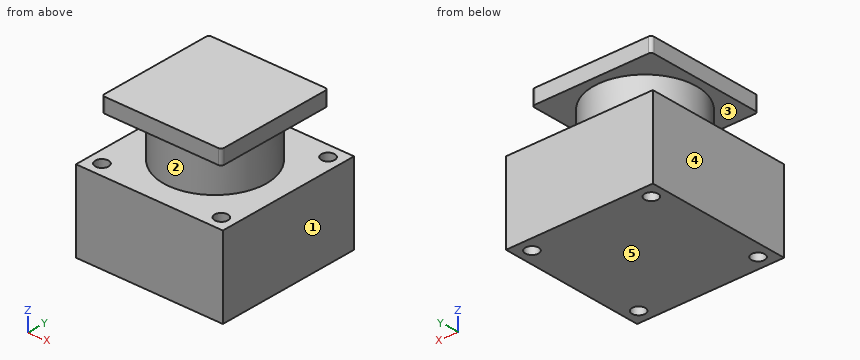
```python
from build123d import *

# Parameters (mm, degrees)
SKETCH_1_W      = 100
SKETCH_1_H      = 100
SKETCH_1_R      = 4.5
EXTRUDE_1_DEPTH = 55
SKETCH_2_R      = 35
EXTRUDE_2_DEPTH = 30
SKETCH_3_W      = 81.317279836
SKETCH_3_H      = 81.317279836
EXTRUDE_3_DEPTH = 10
FILLET_1_R      = 2


with BuildPart() as part:
    # 草图1 → 凸台-拉伸1 (new body)
    with BuildSketch(Plane.XY):
        Rectangle(SKETCH_1_W, SKETCH_1_H)
        with Locations((-40.658639918, 40.658639918)):
            Circle(SKETCH_1_R, mode=Mode.SUBTRACT)
        with Locations((40.658639918, 40.658639918)):
            Circle(SKETCH_1_R, mode=Mode.SUBTRACT)
        with Locations((40.658639918, -40.658639918)):
            Circle(SKETCH_1_R, mode=Mode.SUBTRACT)
        with Locations((-40.658639918, -40.658639918)):
            Circle(SKETCH_1_R, mode=Mode.SUBTRACT)
    extrude(amount=EXTRUDE_1_DEPTH)

    # 草图2 → 凸台-拉伸2 (add)
    with BuildSketch(Plane.XY.offset(55)):
        Circle(SKETCH_2_R)
    extrude(amount=EXTRUDE_2_DEPTH)

    # 草图3 → 凸台-拉伸3 (add)
    with BuildSketch(Plane.XY.offset(85)):
        Rectangle(SKETCH_3_W, SKETCH_3_H)
    extrude(amount=EXTRUDE_3_DEPTH)

    # 圆角1
    fillet_1_edges = [part.edges().sort_by_distance(p)[0] for p in [
        (40.658639918, -40.658639918, 90),
        (40.658639918, 40.658639918, 90),
        (-40.658639918, 40.658639918, 90),
        (-40.658639918, -40.658639918, 90),
    ]]
    fillet(fillet_1_edges, radius=FILLET_1_R)


solid = part.part
```
Geometry: final body of the model. Coordinates: model frame, mm. Face numbers are marked on the shaded views. A direction names the side the tool comes from. Round coordinates to 2 decimals unless told otherwise and drop trailing zeros. Order: outer loops, then holes, each group sorted by start corner. A loop starts at its lowest first (then second) coordinate and runs counter-clockwise, first axis right, second up. Notation, with made-up numbers: (68.25, 16.5) - (88.25, 16.5) arc R18 cw to (88.25, 38.5) - close; hole circle Ø10 at (-12.75, 17). An arc over 180 degrees is marked (long way). Write item = value, one per line. Start each with the question number.
Q1. Pin query (flat end, axial travel): pin 1 (5 mm diameter, centred on x = -17, z = 91, fed in from +Y); pin 2 (2 mm diameter, centred on y = -15.5, z = 66, fed in from -X); pin 3 (8 mm diameter, centred on x = -40.66, y = -40.66, fed in from -Z). Return the tip coordinate at first contact, or that it passes through.
Q2. Cut plane C-C on z = 89. Return the cut outline in (x, y).
Q3. Cut plane B-B on x = 0. Return the cut outline in (y, z), and give its area (3 significant figures).
Q4. Cut plane D-D on y = -6. Return the cut outline in (x, z).
Q5. Access query for the marked faces 1 and 2. Directions: +Z, -Z, +X, -X, +Y, -Y. A direction counts if a zero-diameter tool reaches every point of the face in a straight line with its end or side. Return the directions, or none.
Q6. Ray query, line 1 (Z direction, x = -39, y = 33); line 2 (Z direction, x = 8.5, y = -41); line 3 (X direction, y = 41.5, z = 18). Return the intervals inside material, ascending. Write a range as from..to.
Q7. Pull-direction query (Z, two-part tool) for the marked faces 3, 4 and 5; classes: +Z half, -Z half, draft (parallel to the pull), parting line (faces both ways), or undercut.
Q8. Cut plane A-A on z = 16.5. Return the cut outline in (x, y).
Outcome:
q1.pin_1 = 40.66
q1.pin_2 = -31.86
q1.pin_3 = 85
q2.outline = (-40.66, -38.66) arc R2 ccw to (-38.66, -40.66) - (38.66, -40.66) arc R2 ccw to (40.66, -38.66) - (40.66, 38.66) arc R2 ccw to (38.66, 40.66) - (-38.66, 40.66) arc R2 ccw to (-40.66, 38.66) - close
q3.outline = (-50, 0) - (50, 0) - (50, 55) - (35, 55) - (35, 85) - (40.66, 85) - (40.66, 95) - (-40.66, 95) - (-40.66, 85) - (-35, 85) - (-35, 55) - (-50, 55) - close
q3.area = 8,410 mm^2
q4.outline = (-50, 0) - (50, 0) - (50, 55) - (34.48, 55) - (34.48, 85) - (40.66, 85) - (40.66, 95) - (-40.66, 95) - (-40.66, 85) - (-34.48, 85) - (-34.48, 55) - (-50, 55) - close
q5.face_1 = +Z, -Z, +X, +Y, -Y
q5.face_2 = none
q6.line_1 = 0..55, 85..95
q6.line_2 = 0..55
q6.line_3 = -50..-45.08, -36.24..36.24, 45.08..50
q7.face_3 = undercut
q7.face_4 = draft
q7.face_5 = -Z half
q8.outline = (-50, -50) - (50, -50) - (50, 50) - (-50, 50) - close; hole circle Ø9 at (-40.66, -40.66); hole circle Ø9 at (-40.66, 40.66); hole circle Ø9 at (40.66, -40.66); hole circle Ø9 at (40.66, 40.66)
